Source: CAD feature listing. Evaluate the final solid. Frame: model axes, mm. A direction names the side the tool comes from. Coordinates: 2 decimals unless noted, no trailing zeros. Loops run counter-clockwise (first coordinate to the right, second up) from the corner with the lowest first, then second, coordinate; pieces in that order, holes last. Notation, with made-up numbers: (70.25, 60.25) - (87.25, 60.25) arc R23 cw to (87.25, 91.25) - close; hole circle Ø1 at (42, 26.25). An arc over 180 degrees is marked (long way). Use CSV: the item, a comma, the result in double quotes. Start each with the question number.
```python
from build123d import *

# Parameters (mm, degrees)
F0_W     = 750
F0_H     = 960
F1_DEPTH = 18
F3_DEPTH = 564
F5_DEPTH = 18
F6_W     = 466
F6_H     = 86
F7_DEPTH = 25
F8_W     = 18
F8_H     = 420


with BuildPart() as f1:
    # F0 (on Right) → F1 (new body)
    with BuildSketch(Plane.YZ):
        with Locations((375, 480)):
            Rectangle(F0_W, F0_H)
    extrude(amount=F1_DEPTH)

    # F2 (on face) → F3 (join)
    with BuildSketch(Plane.YZ.offset(18)):
        Polygon((0, 18), (0, 0), (750, 0), (750, 960), (0, 960), (0, 593), (18, 593), (18, 613.75), (18, 942), (732, 942), (732, 275), (732, 182), (732, 18), (636, 18), align=None)
        Polygon((18, 613.75), (18, 593), (572, 275), (590, 275), (608.1493710692, 275), align=None)
        Polygon((732, 182), (636, 18), (732, 18), align=None)
    extrude(amount=F3_DEPTH)

    # F4 (on face) → F5 (join)
    with BuildSketch(Plane.YZ.offset(582)):
        Polygon((750, 960), (0, 960), (0, 593), (18, 593), (572, 275), (608.1493710692, 275), (18, 613.75), (18, 942), (732, 942), (732, 182), (636, 18), (0, 18), (0, 0), (750, 0), align=None)
        Polygon((18, 593), (0, 593), (0, 18), (636, 18), (732, 182), (732, 942), (18, 942), (18, 613.75), (608.1493710692, 275), (572, 275), align=None)
    extrude(amount=F5_DEPTH)

    # F6 (on face) → F7 (cut)
    with BuildSketch(Plane.XZ):
        with Locations((300, 776.5)):
            Rectangle(F6_W, F6_H)
    extrude(amount=-F7_DEPTH, mode=Mode.SUBTRACT)

    # F8 (on face) → F9 (join, up to the next surface of F1)
    with BuildSketch(Plane.XY.offset(18)):
        with Locations((300, 300)):
            Rectangle(F8_W, F8_H)
    extrude(until=Until.NEXT)


solid = f1.part
```
(1) Section B-B on x = 189.5. Output: boundary loops of the cut face in (y, z), plus the area to 3 significant figures.
(2) Section A-A on z = 255. Output: boundary loops of the cut face in (x, y), plus the area to 3 significant figures.
(3) Ray query, line 1 (X direction, y = 453.5, z = 262); line 2 (Y direction, x = 113, z = 699); line 3 (X direction, y = 597, z = 849). Return the intervals inside material, ascending. Write a range as [from, to].
(4) Section D-D on y = 164.5. Output: boundary loops of the cut face in (x, z), plus the area to 3 significant figures.
(5) Section C-C on z = 863.5. Output: boundary loops of the cut face in (x, y), plus the area to 3 significant figures.
(6) Draft query along Z for faces 4 (the flat face through (296, 370, 0)), 5 (the flat face through (296, 750, 473)), 6 (the flat face through (233.385, 291.122, 436.226)). Return one class per face: released by +Z, released by -Z, zero draft, split by the parting line, or undercut.
(7) Reachability of faces 1 (the flat face through (276, 0, 731)), 2 (the flat face through (18, 361, 486)), 3 (the flat face through (291, 297, 222)) from +Z, -Z, +X, -X, +Y, -Y: full face, straight path, thin tool, end or side. Return the list, or none.
(8) Pin query (flat end, axial travel): pin 1 Ø6 at (x, z) = (311, 166.5) entering from -Y. Return the tip coordinate at first contact, or that it passes through.
Solution:
1,outline,"(0, 0) - (750, 0) - (750, 960) - (0, 960) - (0, 819.5) - (18, 819.5) - (18, 942) - (732, 942) - (732, 182) - (636, 18) - (0, 18) - close; (0, 593) - (18, 593) - (572, 275) - (608.15, 275) - (18, 613.75) - (18, 733.5) - (0, 733.5) - close"
1,area,"68,100 mm²"
2,outline,"(0, 0) - (18, 0) - (18, 732) - (582, 732) - (582, 0) - (600, 0) - (600, 750) - (0, 750) - close; (291, 90) - (309, 90) - (309, 510) - (291, 510) - close"
2,area,"44,700 mm²"
3,line 1,"x = [0, 18], [291, 309], [582, 600]"
3,line 2,"y = [0, 18], [732, 750]"
3,line 3,"x = [0, 18], [582, 600]"
4,outline,"(0, 0) - (600, 0) - (600, 960) - (0, 960) - close; hole (18, 18) - (291, 18) - (291, 508.91) - (18, 508.91) - close; hole (18, 529.66) - (582, 529.66) - (582, 942) - (18, 942) - close; hole (309, 18) - (582, 18) - (582, 508.91) - (309, 508.91) - close"
4,area,"75,400 mm²"
5,outline,"(0, 0) - (600, 0) - (600, 750) - (0, 750) - close; hole (18, 18) - (582, 18) - (582, 732) - (18, 732) - close"
5,area,"47,300 mm²"
6,face 4,"released by -Z"
6,face 5,"zero draft"
6,face 6,"undercut"
7,face 1,"+Z, -Z, +X, -X, -Y"
7,face 2,"none"
7,face 3,"-Y"
8,pin 1,"stops at y = 90"
